Model file for the job. Use its own axes, mm. A direction names the side the tool comes from. Give positions to 0.01 mm unless a question says otherwise; leave off trailing zeros. Write each loop counter-clockwise with the first axis right and the second up, starting at its lowest first coordinate (ties: lowest second). Pieces come first, ordered by that corner, then holes. Notation, with made-up numbers: M 20.5,-3 L 29.5,-3 A14 ccw 29.5,16 Z; hole C 76.5,-14.75 d6. An arc over 180 degrees is marked long. Answer as a JSON object with one key per item and string values. Group by question number.
```python
from build123d import *

# Parameters (mm, degrees)
F1_DEPTH = 125
F3_DEPTH = 20.001


with BuildPart() as f1:
    # F0 (on Front) → F1 (new body, symmetric)
    with BuildSketch(Plane.XZ):
        Polygon((0, 20), (0, 0), (20, 0), (20, 2), (2, 2), (2, 20), align=None)
    extrude(amount=F1_DEPTH, both=True)

    # F2 (on face) → F3 (cut, through all)
    with BuildSketch(Plane(origin=(0, 0, 0), x_dir=(0, -1, 0), z_dir=(-1, 0, 0))):
        Polygon((-125, 20), (-125, 0), (-105, 20), align=None)
        Polygon((125, 0), (125, 20), (105, 20), align=None)
    extrude(amount=-F3_DEPTH, mode=Mode.SUBTRACT)


with BuildPart() as f4_1:
    # F4: copy of F1
    add(f1.part)


solid = f4_1.part
```
Q1. 3-axis set-ups, long thin cutter, end or side, ignore diameter. For faces 1 (the flat face through (1.8, 119.5, 5.5)), 2 (the flat face through (2, -2, 11)): which of +Z, -Z, +X, -X, +Y, -Y reach the whole face in a straight line?
Q2. Slice it at A-A, the plane z = 7.25. Write the cut outline in (x, y), then the cut area to 3 significant figures.
Q3. Slice it at B-B, the plane y = 101.5. Write the cut outline in (x, z), then the cut area to 3 significant figures.
Q4. Slice it at C-C, the plane x = 17.5. Write the cut outline in (y, z).
Q5. Drop flat-ended pins along their axis: P1, Ø5.5, axis at x = 9.5, y = 18.5, coming from the +Z side; P2, Ø5, axis at x = 3.5, z = 11, coming from the +Y side; P3, Ø5, axis at y = 48.5, z = 11, coming from the +X side; P4, Ø5, axis at x = 5, z = 16, coming from the -Y side. Give the stop position or say it passes through.
Q6. Wall check: L1, parallel to X at y = 111, z = 4.25; L2, parallel to Y at x = 15, z = 1. Give the ranges that are in metal, low to high.
Solved:
{
 "1": {"face 1": "+Z, +X, -X, +Y", "face 2": "+Z, +X, +Y, -Y"},
 "2": {"outline": "M 0,-117.75 L 2,-117.75 L 2,117.75 L 0,117.75 Z", "area": "471 mm²"},
 "3": {"outline": "M 0,0 L 20,0 L 20,2 L 2,2 L 2,20 L 0,20 Z", "area": "76.0 mm²"},
 "4": {"outline": "M -125,0 L 125,0 L 123,2 L -123,2 Z"},
 "5": {"P1": "stops at z = 2", "P2": "stops at y = 116", "P3": "stops at x = 2", "P4": "passes through"},
 "6": {"L1": "x = 0 to 2", "L2": "y = -124 to 124"}
}
